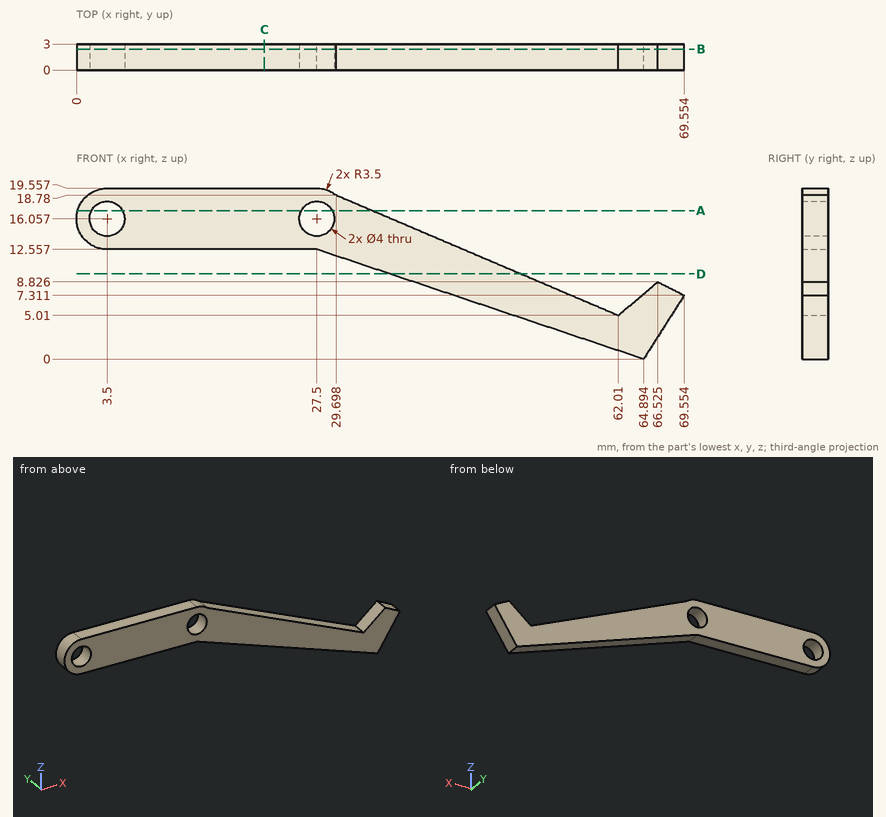
Verification items for this drawing (mm, ordinates from the low corner). Round coordinates to 2 decimals unless told otherwise and drop trailing zeros. Write each loop counter-clockwise with the first axis right and the second up, starting at its lowest first coordinate (ties: lowest second). Pieces come first, ordered by that corner, then holes. Notation, with made-up numbers: (-40, 38) - (-16, 38) arc R23 ccw to (-16, 55) - close; hole circle Ø10 at (81, 49.5). An arc over 180 degrees is marked (long way). One line per item, written item: value.
1. Cross-section at D-D on z = 9.75. Record the boundary of the cut face in (x, y), and give its area (3 significant figures).
The answers:
outline: (35.86, 0) - (50.89, 0) - (50.89, 3) - (35.86, 3) - close
area: 45.1 mm^2
2. Cross-section at B-B on y = 2.4. Record the boundary of the cut face in (x, z) (1 decimal), and give its area (3 significant figures).
The answers:
outline: (3.5, 12.6) - (27.5, 12.6) - (64.9, 0) - (69.6, 7.3) - (66.5, 8.8) - (62, 5) - (29.7, 18.8) arc R3.5 ccw to (27.5, 19.6) - (3.5, 19.6) arc R3.5 ccw to start; hole circle Ø4 at (3.5, 16.1); hole circle Ø4 at (27.5, 16.1)
area: 393 mm^2
3. Scan lines: L1, parallel to Z at x = 28, y = 0.6; L2, parallel to Z at x = 11, y = 0.5; L3, parallel to X at y = 2.8, z = 13.75 (1 decimal). Record each from-to range of solid material in increasing order.
The answers:
L1: z = 12.39 to 14.12, 17.99 to 19.52
L2: z = 12.56 to 19.56
L3: x = 0.9 to 41.5
4. Depth check by flat-ended pin: pin 1 Ø1.5 at (x, y) = (30, 2) entering from +Z; pin 2 Ø3.5 at (x, z) = (3.5, 16.06) entering from -Y. Enter the tip coordinate at first touch or a pass-through.
The answers:
pin 1: stops at z = 19.09
pin 2: passes through
5. Cross-section at A-A on z = 17. Record the boundary of the cut face in (x, y) (1 decimal).
The answers:
outline: (0.1, 0) - (1.7, 0) - (1.7, 3) - (0.1, 3) - close; (5.3, 0) - (25.7, 0) - (25.7, 3) - (5.3, 3) - close; (29.3, 0) - (33.9, 0) - (33.9, 3) - (29.3, 3) - close
6. Cross-section at C-C on x = 21.5. Record the boundary of the cut face in (y, z), and give its area (3 significant figures).
The answers:
outline: (0, 12.56) - (3, 12.56) - (3, 19.56) - (0, 19.56) - close
area: 21.0 mm^2
